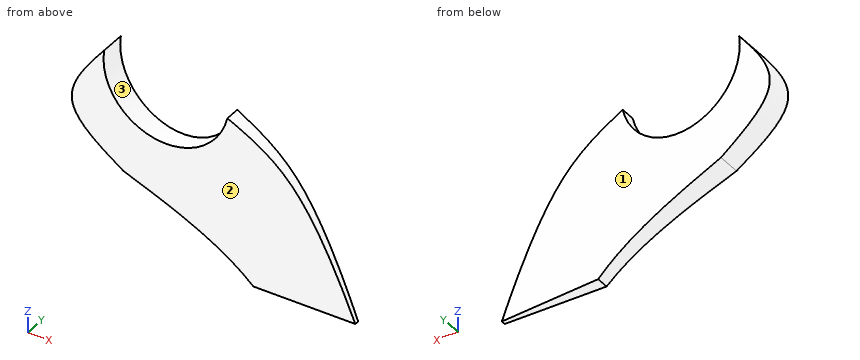
from build123d import *

# Parameters (mm, degrees)
F2_DEPTH = 25.7279276848
F3_DEPTH = 102.7941810931


# Not quite as in the source:
# - a feature names something its author has since deleted; it is built from what else it names


with BuildPart() as f2:
    # F0 (on Front) → F2 (new body, through all)
    with BuildSketch(Plane.XZ):
        with BuildLine():
            ThreePointArc((7.538071066, 90.012077608), (-33.0999025849, 63.2971569556), (-61.4758778659, 102.7931809931))
            add(Edge.make_bspline(
                [(-50.6802275777, 38.4073108435), (-64.2301253741, 47.6853026647), (-91.0055411856, 66.0246371681), (-71.2591028819, 90.6346541889), (-61.4758778659, 102.7931809931)],
                knots=[0, 0, 0, 0, 0.5057307672, 1, 1, 1, 1], degree=3))
            add(Edge.make_bspline(
                [(62.097594142, -64.207687974), (51.1832226367, -40.5716055165), (28.887804967, 7.7111846278), (-23.7900094582, 28.033475615), (-50.6802275777, 38.4073108435)],
                knots=[0, 0, 0, 0, 0.4895343419, 1, 1, 1, 1], degree=3))
            Line((62.097594142, -64.207687974), (96.4130014181, -43.6846762896))
            add(Edge.make_bspline(
                [(96.4130014181, -43.6846762896), (79.9973481318, -1.0988161117), (53.4561883249, 67.712624491), (20.2239489646, 83.857797394), (7.538071066, 90.012077608)],
                knots=[0, 0, 0, 0, 0.6187491541, 1, 1, 1, 1], degree=3))
        make_face()
    extrude(amount=F2_DEPTH)


with BuildPart() as f3:
    # F1 (on Top) → F3 (new body, through all)
    with BuildSketch(Plane.XY):
        Polygon((108.6692065001, -25.7279276848), (-108.6692065001, -7.4702873826), (-108.6692065001, -25.7279276848), align=None)
    extrude(amount=F3_DEPTH)

    # F4: intersect F2
    add(f2.part, mode=Mode.INTERSECT)


solid = f3.part
For this review, take the finished solid that the model builds, in its own axes (mm). Face numbers are marked on the shaded views. Round coordinates to 2 decimals unless told otherwise and drop trailing zeros. Write each question's results on one line, items separated by ' | '. Start each with the question number.
1. Draft analysis for pull direction X (two halves, no side actions). For the marked faces 1, 2 and 3, state which applies: pulls with the +X half, pulls with the -X half, needs draft (parallel to the pull), parting line crosses it, or undercut.
2. Clearance check with flat-ended pins moving along their axes: pin 1 Ø1 at (y, z) = (-20.5, 87.5) entering from +X; pin 2 Ø2 at (y, z) = (-16, 92) entering from -X; pin 3 Ø2 at (x, y) = (-44.5, -15.5) entering from +Z. State where each tip first meets the part, or that it passes through.
3. To check wall thickness, follow L1, parallel to Y at x = 22, z = 11; L2, parallel to X at y = -18.25, z = 90.5; L3, parallel to Y at x = 43, z = 18. State the ranges of each line that lie inside material, in increasing order. Write a range as [from, to].
Output values:
1) face 1: pulls with the +X half | face 2: needs draft | face 3: undercut
2) pin 1: x = 13.68 | pin 2: x = -70.61 | pin 3: z = 68.16
3) L1: [-25.73, -18.45] | L2: [-70.97, -61.05] | L3: [-25.73, -20.21]
